Read the model definition and answer for the solid it produces. Units are mm, in the model's axes. Face numbers are marked on the shaded views. A direction names the side the tool comes from. Give positions to 0.01 mm unless a question says otherwise; leave off trailing zeros. Order: outer loops, then holes, each group sorted by start corner. A loop starts at its lowest first (then second) coordinate and runs counter-clockwise, first axis right, second up.
Item 1: A cutting plane is placed at B-B (x = -6). Write down the section's boundary in (y, z), plus the area to 3 significant figures.
Item 2: Given pin 1 Ø10 at (y, z) = (48.5, 4.5) entering from +X; pin 2 Ø3 at (x, y) = (2, 182.5) entering from +Z; pin 3 Ø8 at (y, z) = (153.5, 0.5) entering from -X, each flat-ended and moving along its own axis, determine where each tip first touches the part or whether it passes through.
Item 3: A cutting plane is placed at C-C (x = 7). Write down the section's boundary in (y, z).
Item 4: Find the intervals of material crossed by line 1 along Y through (x, z) = (6, -0.5); line 2 along X through (y, z) = (225, 2); line 3 along Y through (x, z) = (-1.5, 0.75), in increasing order.
Item 5: Which of the six approach directions +Z, -Z, +X, -X, +Y, -Y give full straight-line access (tool end or side, diameter ignored) to the marked faces 1 and 2?
Item 6: A cutting plane is placed at A-A (y = 112). Write down the section's boundary in (x, z).
from build123d import *

# Parameters (mm, degrees)
SKETCH1_R           = 2.5
BOSS_EXTRUDE1_DEPTH = 254
SKETCH2_R           = 2
BOSS_EXTRUDE2_DEPTH = 10
SKETCH4_R           = 10
BOSS_EXTRUDE3_DEPTH = 5


# Read off the part's stored shape, not the designer's step: M3 Machine Threads Stud1
with BuildPart() as part:
    # Sketch1 → Boss-Extrude1 (new body)
    with BuildSketch(Plane(origin=(0, 0, 0), x_dir=(1, 0, 0), z_dir=(0, 1, 0))):
        with Locations(Location((0, 0, 0), (0, 0, 270))):
            Circle(SKETCH1_R)
    extrude(amount=BOSS_EXTRUDE1_DEPTH)

    # Sketch2 → Boss-Extrude2 (add)
    with BuildSketch(Plane.XZ):
        with Locations(Location((0, 0, 0), (0, 0, 270))):
            Circle(SKETCH2_R)
    extrude(amount=BOSS_EXTRUDE2_DEPTH)

    # M3 Machine Threads Stud1 outline → M3 Machine Threads Stud1 (revolve, cut)
    with BuildSketch(Plane.XY):
        Polygon((2, 0), (1.5, 0), (1.5, -9.7195), (1.2195, -10), (2, -10), align=None)
    revolve(axis=Axis((0, 0, 0), (0, 1, 0)), mode=Mode.SUBTRACT)

    # Sketch4 → Boss-Extrude3 (add)
    with BuildSketch(Plane(origin=(0, 254, 0), x_dir=(1, 0, 0), z_dir=(0, 1, 0))):
        with Locations(Location((0, 0, 0), (0, 0, 270))):
            Circle(SKETCH4_R)
    extrude(amount=BOSS_EXTRUDE3_DEPTH)


solid = part.part
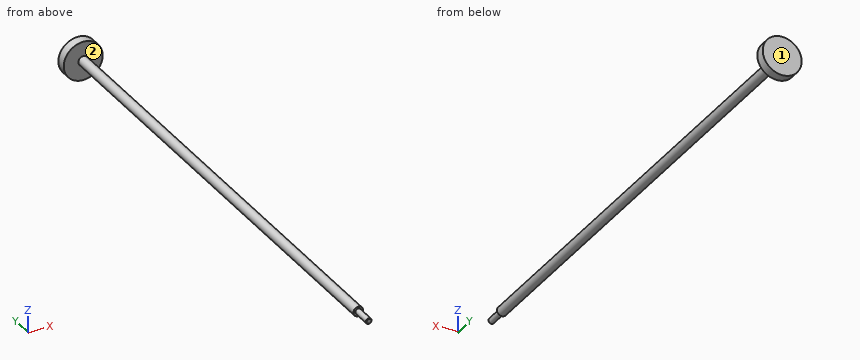
Response values:
1. outline: (254, -8) - (259, -8) - (259, 8) - (254, 8) - close
1. area: 80.0 mm2
2. pin 1: stops at x = 2.5
2. pin 2: stops at z = 2.45
2. pin 3: stops at x = -2.5
3. outline: (254, -7.14) - (259, -7.14) - (259, 7.14) - (254, 7.14) - close
4. line 1: y = 254 to 259
4. line 2: x = -1.5 to 1.5
4. line 3: y = 0 to 259
5. face 1: +Z, -Z, +X, -X, +Y
5. face 2: -Y
6. outline: circle Ø5 at (0, 0)
